Can you work these out from the model? Positions are in its coordinate system, mm. A direction names the side the tool comes from. Round coordinates to 2 decimals unless told otherwise and drop trailing zeros. Order: outer loops, then holes, each group sorted by start corner. A loop starts at its lowest first (then second) coordinate and runs counter-clockwise, first axis right, second up. Notation, with made-up numbers: M -32.75,-33.5 L -5.75,-33.5 A15 cw -5.75,-20.5 Z; hole C 49,45 d9. An arc over 180 degrees is marked long. One line per question, with ' | ' between items.
```python
from build123d import *

# Parameters (mm, degrees)
SKETCH1_R           = 1.5
BOSS_EXTRUDE1_DEPTH = 15
BOSS_EXTRUDE2_DEPTH = 2
BOSS_EXTRUDE3_START = 5
SKETCH3_R           = 1.5
BOSS_EXTRUDE3_DEPTH = 5


with BuildPart() as part:
    # Sketch1 → Boss-Extrude1 (new body)
    with BuildSketch(Plane(origin=(0, 0, 0), x_dir=(1, 0, 0), z_dir=(0, 1, 0))):
        Polygon((3, 0), (1.5, 2.598076211), (-1.5, 2.598076211), (-3, 0), (-1.5, -2.598076211), (1.5, -2.598076211), align=None)
        with Locations(Location((0, 0, 0), (0, 0, 270))):
            Circle(SKETCH1_R, mode=Mode.SUBTRACT)
    extrude(amount=BOSS_EXTRUDE1_DEPTH)

    # Sketch2 → Boss-Extrude2 (add)
    with BuildSketch(Plane.XZ):
        Polygon((1.5, 2.598076211), (-1.5, 2.598076211), (-3, 0), (-1.5, -2.598076211), (1.5, -2.598076211), (3, 0), align=None)
    extrude(amount=BOSS_EXTRUDE2_DEPTH)

    # Sketch3 → Boss-Extrude3 (add)
    with BuildSketch(Plane.XZ.offset(2).offset(BOSS_EXTRUDE3_START)):
        with Locations(Location((0, 0, 0), (0, 0, 90))):
            Circle(SKETCH3_R)
    extrude(amount=-BOSS_EXTRUDE3_DEPTH)


solid = part.part
```
(1) If we section it at A-A on x = 0: Please give me the cut outline in (y, z), plus the area to 3 significant figures.
Final values:
outline: M -7,-1.5 L -2,-1.5 L -2,-2.6 L 15,-2.6 L 15,-1.5 L 0,-1.5 L 0,1.5 L 15,1.5 L 15,2.6 L -2,2.6 L -2,1.5 L -7,1.5 Z | area: 58.3 mm^2
(2) If we section it at C-C on z = 1: Please give me the cut outline in (x, y), plus the area to 3 significant figures.
Final values:
outline: M -2.42,-2 L -1.12,-2 L -1.12,-7 L 1.12,-7 L 1.12,-2 L 2.42,-2 L 2.42,15 L 1.12,15 L 1.12,0 L -1.12,0 L -1.12,15 L -2.42,15 Z | area: 60.0 mm^2
(3) Please list where these lines run through material, in increasing order: probe 1 along Z at (x, y) = (0.05, 11.75); probe 2 along Y at (x, z) = (-2.3, -0.7); probe 3 along Z at (x, y) = (-0.95, 4.25). Write a range as [from, to].
Final values:
probe 1: [-2.6, -1.5], [1.5, 2.6] | probe 2: [-2, 15] | probe 3: [-2.6, -1.16], [1.16, 2.6]
(4) Thinking about a two-plate mould opening in X: for faces 4 (the flat face through (-2.26, 6.62, -1.28)), 5 (the flat face through (0, 0, 0)), 6 (the flat face through (2.24, 6.62, -1.32)), which applies, released by +X, released by -X, zero draft, split by the parting line, or undercut?
Final values:
face 4: released by -X | face 5: undercut | face 6: released by +X
(5) On a 3-axis mill with a long thin cutter (end or side, diameter ignored), from which of +Z, -Z, +X, -X, +Y, -Y can I reach the whole of each face in a straight line? I mean faces 1 (the flat face through (1.3, -2, 1.2)), 2 (the cylindrical face through (0.45, 7.4, 1.43)), 3 (the flat face through (0, -7, 0)). Say none if no direction works.
Final values:
face 1: -Y | face 2: +Y | face 3: +Z, -Z, +X, -X, -Y
(6) If we section it at D-D on y = -2.5: Please give me the cut outline in (x, z), plus the area to 3 significant figures.
Final values:
outline: C 0,0 d3 | area: 7.07 mm^2
(7) Will these pins go through, and if not, where does the flat tip stop? pin 1 Ø1 at (y, z) = (-4, 1.5) entering from +X; pin 2 Ø1.5 at (y, z) = (11, -1.5) entering from -X; pin 3 Ø1 at (y, z) = (11, 1.5) entering from +X.
Final values:
pin 1: x = 1.12 | pin 2: x = -2.57 | pin 3: x = 2.42
(8) If we section it at B-B on y = 3.75: Please give me the cut outline in (x, z).
Final values:
outline: M -3,0 L -1.5,-2.6 L 1.5,-2.6 L 3,0 L 1.5,2.6 L -1.5,2.6 Z; hole C 0,0 d3
